Verification items for this drawing (mm, ordinates from the low corner). Give positions to 0.01 mm unless a question says otherwise; leave off trailing zeros. Order: outer loops, then holes, each group sorted by start corner. A loop starts at its lowest first (then second) coordinate and runs counter-clockwise, first axis right, second up. Notation, with made-up numbers: M 72.5,69 L 106.5,69 A12 cw 106.5,78 Z; hole C 84,7 d5. An arc over 180 degrees is marked long. Answer as a JSON object with one key per item and string values.
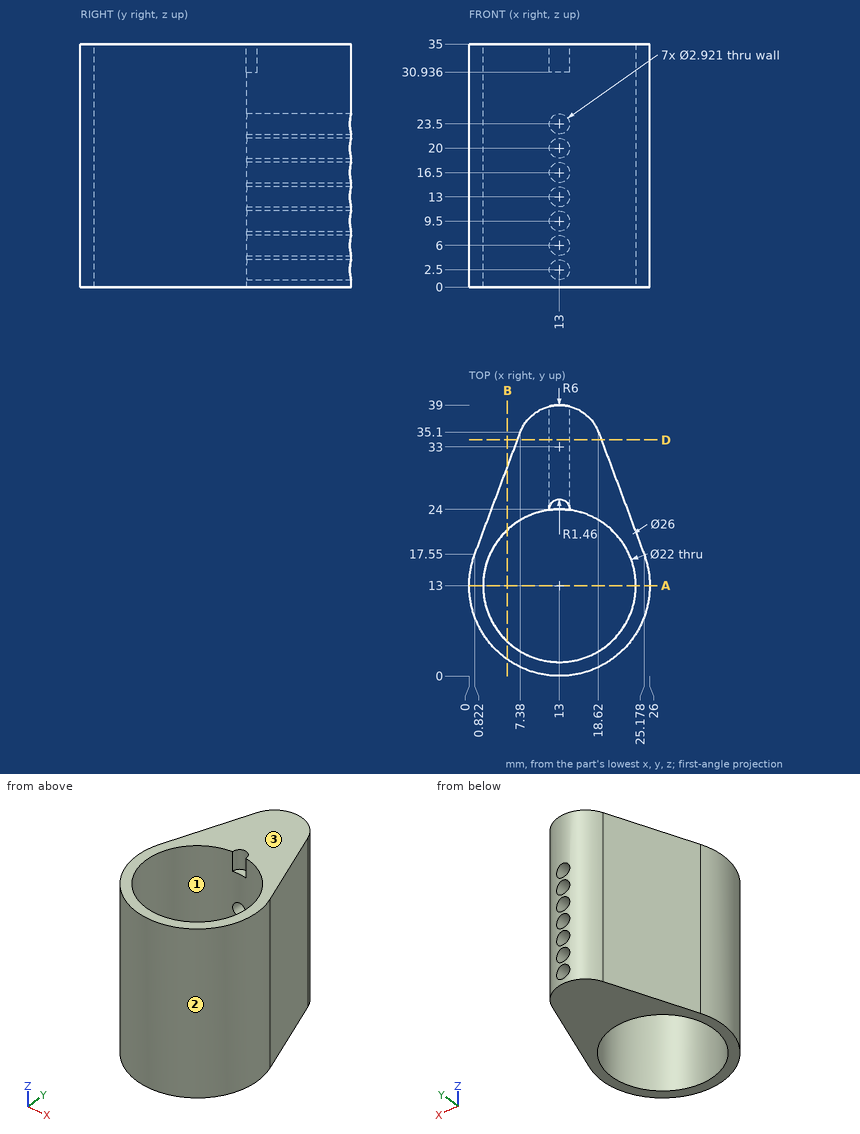
Q1. Section check B-B on x = 5.5. Record the cut outline in (y, z).
Resolved:
{"outline": "M 2.38,0 L 4.95,0 L 4.95,35 L 2.38,35 Z; M 21.05,0 L 30.07,0 L 30.07,35 L 21.05,35 Z"}
Q2. Gauge pin test, flat end, axial feed: pin 1 Ø1.5 at (y, z) = (27, 21.5) entering from +X. Record the tip position at first contact, or that the pin passes through.
Resolved:
{"pin 1": "stops at x = 21.93"}
Q3. Release check for a two-part mould opening along Y. For the marked faces 1, 2 and 3 record: +Y half, -Y half, draft (parallel to the pull), parting line (faces both ways), or undercut.
Resolved:
{"face 1": "undercut", "face 2": "parting line", "face 3": "draft"}
Q4. Section check D-D on y = 34. Record the cut outline in (x, z).
Resolved:
{"outline": "M 6.97,0 L 19.03,0 L 19.03,35 L 6.97,35 Z; hole C 13,2.5 d2.92; hole C 13,6 d2.92; hole C 13,9.5 d2.92; hole C 13,13 d2.92; hole C 13,16.5 d2.92; hole C 13,20 d2.92; hole C 13,23.5 d2.92"}
Q5. Section check A-A on y = 13. Record the cut outline in (x, z), then the cut area to 3 significant figures.
Resolved:
{"outline": "M 0,0 L 2,0 L 2,35 L 0,35 Z; M 24,0 L 26,0 L 26,35 L 24,35 Z", "area": "140 mm²"}
Q6. Material ranges on L1, parallel to X at y = 35, z = 23.5; L2, parallel to Y at x = 9.5, z = 2 (1 decimal); L3, parallel to Y at x = 16.25, z = 30 (1 decimal), recorded low to high.
Resolved:
{"L1": "x = 7.34 to 11.54, 14.46 to 18.66", "L2": "y = 0.5 to 2.6, 23.4 to 37.9", "L3": "y = 0.4 to 2.5, 23.5 to 38"}
